from build123d import *

# Parameters (mm, degrees)
MOTOR_CLAMP_OUTLINE_SOLID_DEPTH     = 7.5
MOTOR_CLAMP_MOUNTING_HOLES_SKETCH_R = 2.25
MOTOR_CLAMP_MOUNTING_HOLE_CUT_DEPTH = 24.532225245


with BuildPart() as part:
    # Motor Clamp Outline Sketch → Motor Clamp Outline Solid (new, symmetric)
    with BuildSketch(Plane.XY):
        with BuildLine():
            Line((-20, 0.125), (-9.999218719, 0.125))
            ThreePointArc((-9.999218719, 0.125), (-9.088484887, 4.171263892), (-6.614378278, 7.5))
            Line((-6.614378278, 7.5), (6.614378278, 7.5))
            ThreePointArc((6.614378278, 7.5), (9.088484887, 4.171263892), (9.999218719, 0.125))
            Line((9.999218719, 0.125), (20, 0.125))
            Line((20, 0.125), (20, 10))
            Line((20, 10), (-20, 10))
            Line((-20, 10), (-20, 0.125))
        make_face()
    extrude(amount=MOTOR_CLAMP_OUTLINE_SOLID_DEPTH, both=True)

    # Motor Clamp Mounting Holes Sketch → Motor Clamp Mounting Hole Cut (cut, through all)
    with BuildSketch(Plane(origin=(0, 10, 0), x_dir=(1, 0, 0), z_dir=(0, 1, 0))):
        with Locations(Location((-15, 0, 0), (0, 0, 270))):
            Circle(MOTOR_CLAMP_MOUNTING_HOLES_SKETCH_R)
        with Locations(Location((15, 0, 0), (0, 0, 270))):
            Circle(MOTOR_CLAMP_MOUNTING_HOLES_SKETCH_R)
    extrude(amount=-MOTOR_CLAMP_MOUNTING_HOLE_CUT_DEPTH, mode=Mode.SUBTRACT)


solid = part.part
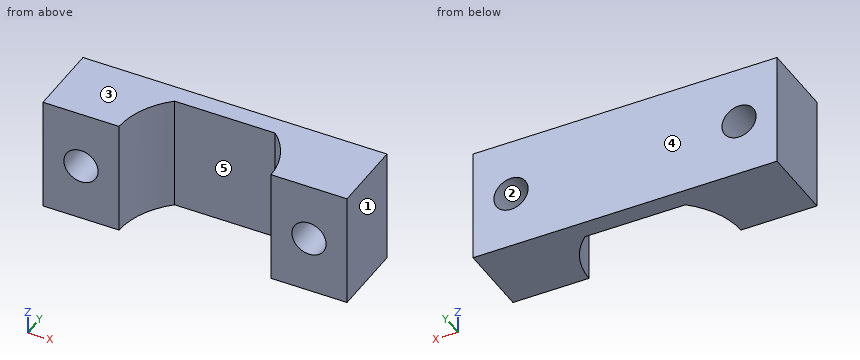
Design review of the part built by this model. Coordinates are the model's own, in mm. Face numbers are marked on the shaded views. A direction names the side the tool comes from. Give positions to 0.01 mm unless a question says otherwise; leave off trailing zeros. Order: outer loops, then holes, each group sorted by start corner. A loop starts at its lowest first (then second) coordinate and runs counter-clockwise, first axis right, second up. Notation, with made-up numbers: (-11.75, -26) - (-3.75, -26) arc R18 ccw to (-3.75, -8) - close; hole circle Ø3 at (64.5, 25). An arc over 180 degrees is marked (long way). Write item = value, one per line. Start each with the question number.
Q1. To check wall thickness, follow L1, parallel to X at y = 9.5, z = -1.5; L2, parallel to X at y = 5.75, z = 0; L3, parallel to X at y = 5, z = 0. State the ranges of each line that lie inside material, in increasing order. Write a range as from..to.
Q2. Clearance check with flat-ended pins moving along their axes: pin 1 Ø6.5 at (x, z) = (-3, -1) entering from -Y; pin 2 Ø2.5 at (x, z) = (-15, 0) entering from -Y. State where each tip first meets the part, or that it passes through.
Q3. Mouldability with a two-part tool opening along Z and no side actions: class the marked faces 1, 2 and 3 as released by +Z, released by -Z, zero draft, split by the parting line, or undercut.
Q4. We need section D-D on z = 4.5. State the section outline as (x, y) points (3 decimals), plus the area to 3 significant figures.
Q5. Tool access review of the marked faces 4 and 5: name each direction out of +Z, -Z, +X, -X, +Y, -Y from which nothing blocks a thin tool from reaching the whole face with its end or side.
Q6. We need section A-A on z = 0. State the section outline as (x, y) points (3 decimals), plus the area to 3 significant figures.
Q7. We need section C-C on y = 7. State the section outline as (x, z) points.
Q8. We need section B-B on x = 15. State the section outline as (y, z) points (3 decimals).
Working result:
q1.L1 = -20..-16.68, -13.32..13.32, 16.68..20
q1.L2 = -20..-17.25, -12.75..-8.18, 8.18..12.75, 17.25..20
q1.L3 = -20..-17.25, -12.75..-8.66, 8.66..12.75, 17.25..20
q2.pin_1 = 7.5
q2.pin_2 = through
q3.face_1 = zero draft
q3.face_2 = undercut
q3.face_3 = released by +Z
q4.outline = (-20, 0.125) - (-9.999, 0.125) arc R10 cw to (-6.614, 7.5) - (6.614, 7.5) arc R10 cw to (9.999, 0.125) - (20, 0.125) - (20, 10) - (-20, 10) - close
q4.area = 263 mm²
q5.face_4 = +Z, -Z, +X, -X, +Y
q5.face_5 = +Z, -Z, -Y
q6.outline = (-20, 0.125) - (-17.25, 0.125) - (-17.25, 10) - (-20, 10) - close; (-12.75, 0.125) - (-9.999, 0.125) arc R10 cw to (-6.614, 7.5) - (6.614, 7.5) arc R10 cw to (9.999, 0.125) - (12.75, 0.125) - (12.75, 10) - (-12.75, 10) - close; (17.25, 0.125) - (20, 0.125) - (20, 10) - (17.25, 10) - close
q6.area = 174 mm²
q7.outline = (-20, -7.5) - (-7.14, -7.5) - (-7.14, 7.5) - (-20, 7.5) - close; (7.14, -7.5) - (20, -7.5) - (20, 7.5) - (7.14, 7.5) - close; hole circle Ø4.5 at (-15, 0); hole circle Ø4.5 at (15, 0)
q8.outline = (0.125, -7.5) - (10, -7.5) - (10, -2.25) - (0.125, -2.25) - close; (0.125, 2.25) - (10, 2.25) - (10, 7.5) - (0.125, 7.5) - close
